```python
from build123d import *

# Parameters (mm, degrees)
F1_DEPTH      = 11.4
F3_DEPTH      = 25
F5_DEPTH      = 12.5
F7_DEPTH      = 3.62
F9_DEPTH      = 25
F9_DEPTH_BACK = 49.7


with BuildPart() as f1:
    # F0 (on Top) → F1 (new body)
    with BuildSketch(Plane.XY):
        with BuildLine():
            Line((0, 21.6441951712), (18.1235127774, 0))
            Line((18.1235127774, 0), (18.4301963788, 0.256797914))
            Line((18.4301963788, 0.256797914), (0.3066836014, 21.9009930852))
            ThreePointArc((0.3066836014, 21.9009930852), (-3.986202338, 25.1744521896), (-9.269486464, 26.2840976478))
            Line((-9.269486464, 26.2840976478), (-23.1229464174, 25.8354809233))
            Line((-23.1229464174, 25.8354809233), (-23.11, 25.4356904904))
            Line((-23.11, 25.4356904904), (-9.26, 25.8841951712))
            ThreePointArc((-9.26, 25.8841951712), (-4.1511288202, 24.8100317574), (0, 21.6441951712))
        make_face()
        Polygon((-23.1229464174, 25.8354809233), (-9.269486464, 26.2840976478), (-9.2840532536, 26.7339258093), (-23.1267969944, 26.285656108), align=None)
    extrude(amount=F1_DEPTH)

    # F2 (on face) → F3 (cut)
    with BuildSketch(Plane(origin=(10.6537746153, 8.9208131252, 0), x_dir=(0.6419947849, -0.7667090036, 0), z_dir=(-0.7667090036, -0.6419947849, 0))):
        Polygon((-16.5947993131, 4.18), (11.6352006869, 1.35), (11.6352006869, 11.4), (-16.5947993131, 11.4), align=None)
    extrude(amount=-F3_DEPTH, mode=Mode.SUBTRACT)

    # F4 (on face) → F5 (cut, symmetric)
    with BuildSketch(Plane(origin=(-0.8470304755, 26.1566324428, 0), x_dir=(0.9994760824, 0.0323660434, 0), z_dir=(0.0323660434, -0.9994760824, 0))):
        Polygon((-22.2746396009, 7.5215270421), (-21.4173795381, 7.38), (-21.4173795381, 11.4), (-22.2746396009, 11.4), align=None)
        Polygon((-21.4173795381, 7.38), (-8.4173795381, 5.2338), (-8.4173795381, 11.4), (-21.4173795381, 11.4), align=None)
        Polygon((-8.4173795381, 11.4), (-8.4173795381, 5.2338), (0.7005369606, 4.18), (0.7005369606, 11.4), align=None)
        Polygon((0.7005369606, 11.4), (0.7005369606, 4.18), (18.1140175495, 1.35), (18.1140175495, 8.57), (18.1140175495, 11.4), align=None)
    extrude(amount=F5_DEPTH, both=True, mode=Mode.SUBTRACT)

    # F6 (on face) → F7 (join)
    with BuildSketch(Plane(origin=(-0.8470304755, 26.1566324428, 0), x_dir=(0.9994760824, 0.0323660434, 0), z_dir=(0.0323660434, -0.9994760824, 0))):
        Polygon((-22.2746396009, 7.5215270421), (-22.2746396009, 0), (-21.4246396009, 0), (-21.4246396009, 7.3811985805), align=None)
    extrude(amount=F7_DEPTH)

    # F8 (on face) → F9 (cut, two sides)
    with BuildSketch(Plane(origin=(-0.8470304755, 26.1566324428, 0), x_dir=(0.9994760824, 0.0323660434, 0), z_dir=(0.0323660434, -0.9994760824, 0))) as f9_sk:
        Polygon((-8.4173795381, 5.2338), (-8.4173795381, 0), (-8.4173795381, -8.5982028395), (53.2149014449, -45.262684235), (51.573908383, 51.0224351168), (-8.4173795381, 50), align=None)
    extrude(amount=-F9_DEPTH, mode=Mode.SUBTRACT)
    extrude(f9_sk.sketch, amount=F9_DEPTH_BACK, mode=Mode.SUBTRACT)


solid = f1.part
```
Read the model definition and answer for the solid it produces. Units are mm, in the model's axes. Give positions to 0.01 mm unless a question says otherwise; leave off trailing zeros. Write each loop counter-clockwise with the first axis right and the second up, starting at its lowest first coordinate (ties: lowest second). Pieces come first, ordered by that corner, then holes. Notation, with made-up numbers: (-26.75, 31.5) - (-4.75, 31.5) arc R28 cw to (-4.75, 60.5) - close; hole circle Ø10 at (-30, 89.5). An arc over 180 degrees is marked (long way). Write item = value, one per line. Start each with the question number.
Item 1: Find the intervals of material crossed by probe 1 along X at (y, z) = (25.95, 5); probe 2 along Y at (x, z) = (-13.5, 0.75); probe 3 along X at (y, z) = (24.5, 7), in increasing order. Write a range as [from, to].
Item 2: Each of these flat-tipped pins is pushed along its axis until it touches: P1, Ø1.5, axis at x = -12, z = 3.5, coming from the -Y side; P2, Ø1.5, axis at x = -18, y = 26, coming from the +Z side. Where does it stop, or does it pass through?
Item 3: Find section D-D (z = 5.5). Give the vertices of the cut face in (x, y), then the cut area to 3 significant figures.
Item 4: Find section C-C (x = -15.25). Give the vertices of the cut face in (y, z), then the cut area to 3 significant figures.
Item 5: Find section A-A (z = 4). Give the vertices of the cut face in (x, y).
Item 6: Find section B-B (y = 25.7). Give the vertices of the cut face in (x, z), then the cut area to 3 significant figures.
Response:
q1.probe_1 = [-23.12, -9.26]
q1.probe_2 = [25.75, 26.6]
q1.probe_3 = [-23.08, -22.23]
q2.P1 = 25.77
q2.P2 = 6.8
q3.outline = (-23.13, 26.29) - (-23.12, 25.84) - (-22.99, 21.82) - (-22.14, 21.85) - (-22.26, 25.46) - (-10.87, 25.83) - (-10.9, 26.68) - close
q3.area = 13.5 mm²
q4.outline = (25.69, 0) - (26.54, 0) - (26.54, 6.22) - (25.69, 6.22) - close
q4.area = 5.29 mm²
q5.outline = (-23.13, 26.29) - (-23.12, 25.84) - (-22.99, 21.82) - (-22.14, 21.85) - (-22.26, 25.46) - (-9.26, 25.88) - (-9.29, 26.73) - close
q6.outline = (-23.12, 0) - (-14.95, 0) - (-14.95, 6.17) - (-23.12, 7.52) - close
q6.area = 55.9 mm²
